from build123d import *

# Parameters (mm, degrees)
F0_R     = 1.75
F0_R_2   = 51.75
F1_DEPTH = 15


# Not quite as in the source:
# - ends of sketch curves that miss each other by under 0.0002 mm in the source are joined


with BuildPart() as f1:
    # F0 (on Right) → F1 (new body)
    with BuildSketch(Plane.YZ):
        Polygon((-59.9995488366, -115.0645988089), (60.0004511634, -115.0645988089), (60.0004498223, 124.9354011911), (0.0004538456, 124.9354011911), (-59.9995488366, 124.9354011911), align=None)
        with Locations((-49.9999973178, -107.0645988089)):
            Circle(F0_R, mode=Mode.SUBTRACT)
        with Locations((-40.3050865276, -73.1196853366)):
            Circle(F0_R, mode=Mode.SUBTRACT)
        with Locations((0.0004511634, -32.8145988089)):
            Circle(F0_R_2, mode=Mode.SUBTRACT)
        with Locations((50.0000026822, -107.0645988089)):
            Circle(F0_R, mode=Mode.SUBTRACT)
        with Locations((40.3050865276, -73.1196853366)):
            Circle(F0_R, mode=Mode.SUBTRACT)
        with Locations((-40.3050865276, 7.4904877187)):
            Circle(F0_R, mode=Mode.SUBTRACT)
        with Locations((-49.9995488366, 116.9354011911)):
            Circle(F0_R, mode=Mode.SUBTRACT)
        with Locations((40.305537691, 7.4904877187)):
            Circle(F0_R, mode=Mode.SUBTRACT)
        with BuildLine():
            Line((-19.4991003554, 110.9354010969), (19.5008996446, 110.9354010969))
            ThreePointArc((19.5008996446, 110.9354010969), (23.3899869411, 109.3244883935), (25.0008996446, 105.4354010969))
            Line((25.0008996446, 105.4354010969), (25.0008996446, 36.4354010969))
            ThreePointArc((25.0008996446, 36.4354010969), (23.3899869411, 32.5463138004), (19.5008996446, 30.9354010969))
            Line((19.5008996446, 30.9354010969), (-19.4991003554, 30.9354010969))
            ThreePointArc((-19.4991003554, 30.9354010969), (-23.3881876519, 32.5463138004), (-24.9991003554, 36.4354010969))
            Line((-24.9991003554, 36.4354010969), (-24.9991003554, 105.4354010969))
            ThreePointArc((-24.9991003554, 105.4354010969), (-23.3881876519, 109.3244883935), (-19.4991003554, 110.9354010969))
        make_face(mode=Mode.SUBTRACT)
        with Locations((50.0004511634, 116.9354046481)):
            Circle(F0_R, mode=Mode.SUBTRACT)
    extrude(amount=-F1_DEPTH)


solid = f1.part
Design review of the part built by this model. Coordinates are the model's own, in mm. A direction names the side the tool comes from. Round coordinates to 2 decimals unless told otherwise and drop trailing zeros. Loops run counter-clockwise (first coordinate to the right, second up) from the corner with the lowest first, then second, coordinate; pieces in that order, holes last. Notation, with made-up numbers: M 9,47 L 16,47 A24 cw 16,70 Z; hole C 3.25,26.25 d4. An arc over 180 degrees is marked long. Answer as a JSON object with one key per item and string values.
Item 1: We need section C-C on x = -4. State how many separate pieces and enclosed holes the cut face has, and give its area (3 significant figures).
Answer sheet:
{"separate pieces": "1", "enclosed holes": "10", "area": "16,300 mm^2"}
Item 2: We need section D-D on y = 6.5. Give the boundary of the cut face in (x, z).
Answer sheet:
{"outline": "M -15,-115.06 L 0,-115.06 L 0,-84.15 L -15,-84.15 Z; M -15,18.53 L 0,18.53 L 0,30.94 L -15,30.94 Z; M -15,110.94 L 0,110.94 L 0,124.94 L -15,124.94 Z"}
Item 3: We need section B-B on y = 33. Give the boundary of the cut face in (x, z).
Answer sheet:
{"outline": "M -15,-115.06 L 0,-115.06 L 0,-72.68 L -15,-72.68 Z; M -15,7.05 L 0,7.05 L 0,124.94 L -15,124.94 Z"}
Item 4: The part is to be moulded in two halves that separate along Y. For faces 1 (the flat face through (-7, 0, 30.935)), 2 (the flat face through (-7, 60, 3)), 3 (the flat face through (-7, -60, 7)), say which applies: pulls with the +Y half, pulls with the -Y half, needs draft (parallel to the pull), parting line crosses it, or undercut.
Answer sheet:
{"face 1": "undercut", "face 2": "pulls with the +Y half", "face 3": "pulls with the -Y half"}
Item 5: Clearance check with a flat-ended pin moving along its axis: P1, Ø4.5, axis at y = 50, z = -107.06, coming from the +X side. State where the tip first meets the part, or that it passes through.
Answer sheet:
{"P1": "stops at x = 0"}
Item 6: Machinability: for faces 4 (the flat face through (-7, 25.001, 71)), 5 (the flat face through (-7, -1, -115.065)), which of the approach directions +Z, -Z, +X, -X, +Y, -Y give a long, thin tool a straight path to every point of the face, cutting with its end or side? Answer none if there is none.
Answer sheet:
{"face 4": "+X, -X", "face 5": "-Z, +X, -X, +Y, -Y"}
Item 7: Wall thickness on L1, parallel to Y at x = -12.25, z = 62.5; L2, parallel to Z at x = -1.25, y = 39.5; L3, parallel to Z at x = -1.5, y = -18.5: over which ranges is each line inside the solid? List them lowest first. Write a range as from..to.
Answer sheet:
{"L1": "y = -60..-25, 25..60", "L2": "z = -115.06..-74.67, -71.57..-66.25, 0.62..5.94, 9.04..124.94", "L3": "z = -115.06..-81.14, 15.52..30.94, 110.94..124.94"}
Item 8: We need section A-A on z = 57. Give the boundary of the cut face in (x, y), and give its area (3 significant figures).
Answer sheet:
{"outline": "M -15,-60 L 0,-60 L 0,-25 L -15,-25 Z; M -15,25 L 0,25 L 0,60 L -15,60 Z", "area": "1,050 mm^2"}
